```python
from build123d import *

# Parameters (mm, degrees)
F1_DEPTH = 20
F2_DEPTH = 12
F3_R     = 3
F4_R     = 2
F6_DEPTH = 3


with BuildPart() as f1:
    # F0 (on Top) → F1 (new body)
    with BuildSketch(Plane.XY):
        with BuildLine():
            Line((-2.7276199649, -5.0460615367), (-9.3815706973, -5.0460615367))
            ThreePointArc((-9.3815706973, -5.0460615367), (-8.3933511583, -7.0038733026), (-7.002121491, -8.6991858936))
            ThreePointArc((-7.002121491, -8.6991858936), (-0.0140736997, -11.5460615367), (6.9739740916, -8.6991858936))
            ThreePointArc((6.9739740916, -8.6991858936), (8.3652037588, -7.0038733026), (9.3534232979, -5.0460615367))
            Line((9.3534232979, -5.0460615367), (2.6994725655, -5.0460615367))
            Line((2.6994725655, -5.0460615367), (2.353062404, -5.6460615367))
            Line((2.353062404, -5.6460615367), (-2.3812098034, -5.6460615367))
            Line((-2.3812098034, -5.6460615367), (-2.7276199649, -5.0460615367))
        make_face()
        with BuildLine():
            Line((-2.7276199649, 1.9539384633), (-9.3815706973, 1.9539384633))
            ThreePointArc((-9.3815706973, 1.9539384633), (-10.0140736997, -1.5460615367), (-9.3815706973, -5.0460615367))
            Line((-9.3815706973, -5.0460615367), (-2.7276199649, -5.0460615367))
            Line((-2.7276199649, -5.0460615367), (-4.7483459071, -1.5460615367))
            Line((-4.7483459071, -1.5460615367), (-2.7276199649, 1.9539384633))
        make_face()
        with BuildLine():
            ThreePointArc((-7.002121491, 5.6070628203), (-8.3933511583, 3.9117502293), (-9.3815706973, 1.9539384633))
            Line((-9.3815706973, 1.9539384633), (-2.7276199649, 1.9539384633))
            Line((-2.7276199649, 1.9539384633), (-2.3812098034, 2.5539384633))
            Line((-2.3812098034, 2.5539384633), (2.353062404, 2.5539384633))
            Line((2.353062404, 2.5539384633), (2.6994725655, 1.9539384633))
            Line((2.6994725655, 1.9539384633), (9.3534232979, 1.9539384633))
            ThreePointArc((9.3534232979, 1.9539384633), (8.3652037588, 3.9117502293), (6.9739740916, 5.6070628203))
            ThreePointArc((6.9739740916, 5.6070628203), (-0.0140736997, 8.4539384633), (-7.002121491, 5.6070628203))
        make_face()
        with BuildLine():
            Line((9.3534232979, 1.9539384633), (2.6994725655, 1.9539384633))
            Line((2.6994725655, 1.9539384633), (4.7201985076, -1.5460615367))
            Line((4.7201985076, -1.5460615367), (2.6994725655, -5.0460615367))
            Line((2.6994725655, -5.0460615367), (9.3534232979, -5.0460615367))
            ThreePointArc((9.3534232979, -5.0460615367), (9.8265301937, -3.3244076818), (9.9859263003, -1.5460615367))
            ThreePointArc((9.9859263003, -1.5460615367), (9.8265301937, 0.2322846085), (9.3534232979, 1.9539384633))
        make_face()
    extrude(amount=F1_DEPTH)

    # F0 (on Top) → F2 (join)
    with BuildSketch(Plane.XY):
        with BuildLine():
            ThreePointArc((9.3534232979, -5.0460615367), (8.3652037588, -7.0038733026), (6.9739740916, -8.6991858936))
            ThreePointArc((6.9739740916, -8.6991858936), (13.2284079346, -5.9766630079), (19.9859263003, -5.0460615367))
            Line((19.9859263003, -5.0460615367), (9.3534232979, -5.0460615367))
        make_face()
        with BuildLine():
            ThreePointArc((19.9859263003, 1.9539384633), (13.2284079346, 2.8845399345), (6.9739740916, 5.6070628203))
            ThreePointArc((6.9739740916, 5.6070628203), (8.3652037588, 3.9117502293), (9.3534232979, 1.9539384633))
            Line((9.3534232979, 1.9539384633), (19.9859263003, 1.9539384633))
        make_face()
        with BuildLine():
            Line((19.9859263003, 1.9539384633), (9.3534232979, 1.9539384633))
            ThreePointArc((9.3534232979, 1.9539384633), (9.8265301937, 0.2322846085), (9.9859263003, -1.5460615367))
            ThreePointArc((9.9859263003, -1.5460615367), (9.8265301937, -3.3244076818), (9.3534232979, -5.0460615367))
            Line((9.3534232979, -5.0460615367), (19.9859263003, -5.0460615367))
            Line((19.9859263003, -5.0460615367), (34.9859263003, -5.0460615367))
            Line((34.9859263003, -5.0460615367), (34.9859263003, 1.9539384633))
            Line((34.9859263003, 1.9539384633), (19.9859263003, 1.9539384633))
        make_face()
        with BuildLine():
            Line((-9.3815706973, -5.0460615367), (-20.0140736997, -5.0460615367))
            ThreePointArc((-20.0140736997, -5.0460615367), (-13.2565553341, -5.9766630079), (-7.002121491, -8.6991858936))
            ThreePointArc((-7.002121491, -8.6991858936), (-8.3933511583, -7.0038733026), (-9.3815706973, -5.0460615367))
        make_face()
        with BuildLine():
            Line((-20.0140736997, 1.9539384633), (-35.0140736997, 1.9539384633))
            Line((-35.0140736997, 1.9539384633), (-35.0140736997, -5.0460615367))
            Line((-35.0140736997, -5.0460615367), (-20.0140736997, -5.0460615367))
            Line((-20.0140736997, -5.0460615367), (-9.3815706973, -5.0460615367))
            ThreePointArc((-9.3815706973, -5.0460615367), (-10.0140736997, -1.5460615367), (-9.3815706973, 1.9539384633))
            Line((-9.3815706973, 1.9539384633), (-20.0140736997, 1.9539384633))
        make_face()
        with BuildLine():
            ThreePointArc((-7.002121491, 5.6070628203), (-13.2565553341, 2.8845399345), (-20.0140736997, 1.9539384633))
            Line((-20.0140736997, 1.9539384633), (-9.3815706973, 1.9539384633))
            ThreePointArc((-9.3815706973, 1.9539384633), (-8.3933511583, 3.9117502293), (-7.002121491, 5.6070628203))
        make_face()
    extrude(amount=F2_DEPTH)

    # F3
    f3_edges = [f1.edges().sort_by_distance(p)[0] for p in [
        (-35.014074, 1.953938, 6),
        (-35.014074, -5.046062, 6),
        (34.985926, -5.046062, 6),
        (34.985926, 1.953938, 6),
    ]]
    fillet(f3_edges, radius=F3_R)

    # F4
    f4_edges = [f1.edges().sort_by_distance(p)[0] for p in [
        (-26.014074, -5.046062, 12),
        (13.228408, -5.976663, 12),
        (-9.381571, 1.953938, 20),
    ]]
    fillet(f4_edges, radius=F4_R)

    # F5 (on Front) → F6 (join)
    with BuildSketch(Plane.XZ):
        with BuildLine():
            ThreePointArc((-9.5652169443, 17.9530884136), (-13.9630221988, 13.5080377527), (-19.999999553, 11.8789058179))
            Line((-19.999999553, 11.8789058179), (-9.5652169443, 11.8789058179))
            Line((-9.5652169443, 11.8789058179), (-9.5652169443, 17.9530884136))
        make_face()
        with BuildLine():
            ThreePointArc((20.000000447, 11.8789058179), (13.9630230929, 13.5080377527), (9.5652178383, 17.9530884136))
            Line((9.5652178383, 17.9530884136), (9.5652178383, 11.8789058179))
            Line((9.5652178383, 11.8789058179), (20.000000447, 11.8789058179))
        make_face()
    extrude(amount=F6_DEPTH)


solid = f1.part
```
Can you work these out from the model? Positions are in its coordinate system, mm. A direction names the side the tool comes from. Coordinates: 2 decimals unless noted, no trailing zeros. Write each loop counter-clockwise with the first axis right and the second up, starting at its lowest first coordinate (ties: lowest second). Pieces come first, ordered by that corner, then holes. Notation, with made-up numbers: (-28, 88) - (23, 88) arc R16 ccw to (23, 117) - close; hole circle Ø4 at (-28.5, -10). An arc over 180 degrees is marked (long way). Return JSON: item names as keys, results as strings.
Q1. Thinking about a two-plate mould opening in Y: for faces 4 (the cylindrical face through (26.07, -4.476, 11.399)), 5 (the flat face through (-1, 3, 0)), 6 (the flat face through (0, 2.554, 10)), which applies, +Y half, -Y half, draft (parallel to the pull), parting line (faces both ways), or undercut?
Computed values:
{"face 4": "-Y half", "face 5": "draft", "face 6": "undercut"}
Q2. I'm going to push flat-ended pins straight in: pin 1 Ø8 at (x, z) = (-26, 6) entering from -Y; pin 2 Ø3.5 at (x, y) = (-23.5, -1.5) entering from +Z; pin 3 Ø6 at (x, z) = (13, 13.5) entering from +Y. Where does each tip first touch, or does it pass through?
Computed values:
{"pin 1": "stops at y = -5.05", "pin 2": "stops at z = 12", "pin 3": "stops at y = 3.21"}
Q3. Please list where these lines run through material, in increasing order: L1, parallel to X at y = 6.75, z = 3.5; L2, parallel to Y at x = -6, z = 13.25; L3, parallel to X at y = -0.75, z = 16.25. Write a range as from..to.
Computed values:
{"L1": "x = -5.6..5.57", "L2": "y = -9.56..6.46", "L3": "x = -10.74..-4.29, 4.26..10.74"}
Q4. If we section it at B-B (x = 28.5): Please give me the cut outline in (y, z), then the cut area to 3 significant figures.
Computed values:
{"outline": "(-5.05, 0) - (1.95, 0) - (1.95, 10) arc R2 ccw to (-0.05, 12) - (-3.05, 12) arc R2 ccw to (-5.05, 10) - close", "area": "82.3 mm2"}
Q5. If we section it at A-A (z = 2.5): Please give me the cut outline in (x, y).
Computed values:
{"outline": "(-35.01, -2.05) arc R3 ccw to (-32.01, -5.05) - (-20.01, -5.05) arc R25 cw to (-7, -8.7) arc R10 ccw to (6.97, -8.7) arc R25 cw to (19.99, -5.05) - (31.99, -5.05) arc R3 ccw to (34.99, -2.05) - (34.99, -1.05) arc R3 ccw to (31.99, 1.95) - (19.99, 1.95) arc R25 cw to (6.97, 5.61) arc R10 ccw to (-7, 5.61) arc R25 cw to (-20.01, 1.95) - (-32.01, 1.95) arc R3 ccw to (-35.01, -1.05) - close; hole (-4.75, -1.55) - (-2.38, -5.65) - (2.35, -5.65) - (4.72, -1.55) - (2.35, 2.55) - (-2.38, 2.55) - close"}
Q6. On a 3-axis mill with a long thin cutter (end or side, diameter ignored), from which of +Z, -Z, +X, -X, +Y, -Y can I reach the whole of each face in a straight line? I mean faces 1 (the cylindrical face through (-25.93, -4.476, 11.399)), 2 (the flat face through (12, 0, 14)), 3 (the flat face through (0, -5.646, 10)). Say none if no direction works.
Computed values:
{"face 1": "+Z, -X, -Y", "face 2": "+Z, +X, +Y", "face 3": "+Z, -Z"}
Q7. If we section it at C-C (z = 16.25): Please give me the cut outline in (x, y).
Computed values:
{"outline": "(-10.74, -3) - (-9.91, -3) arc R10 ccw to (9.88, -3) - (10.74, -3) - (10.74, 0) - (9.87, 0) arc R10 ccw to (-9.89, 0) - (-10.74, 0) - close; hole (-4.75, -1.55) - (-2.38, -5.65) - (2.35, -5.65) - (4.72, -1.55) - (2.35, 2.55) - (-2.38, 2.55) - close"}
